Source: CAD feature listing. Evaluate the final solid. Frame: model axes, mm. A direction names the side the tool comes from. Give positions to 0.01 mm unless a question says otherwise; leave off trailing zeros. Loops run counter-clockwise (first coordinate to the right, second up) from the corner with the lowest first, then second, coordinate; pieces in that order, holes last. Notation, with made-up numbers: (46, 40.5) - (92, 40.5) arc R5 ccw to (92, 45.5) - close; hole circle Ø1 at (59.5, 62). An arc over 180 degrees is marked (long way). Write each question's results on one line, items separated by ' | '. Start each with the question number.
(1) Cut plane B-B on y = -8. Return the cut outline in (x, z).
(2) Contact query for flat-ended pins moving along their axis: pin 1 (2 mm diameter, centred on y = -1, z = -9.5, fed in from -X); pin 2 (5 mm diameter, centred on x = 8.5, z = -1, fed in from -Y); pin 3 (1.5 mm diameter, centred on x = 3, y = -1.5, fed in from +Z); pin 4 (4 mm diameter, centred on x = 3.5, y = -10, fed in from +Z). Output: stop coordinate, or through.
(3) Cut plane D-D on z = -6. Return the cut outline in (x, y).
(4) Reachability of faces 5 (the cylindrical face through (0.8, -0.95, 10.75)), 6 (the cylindrical face through (2.937, 0.056, 12.834)) from +Z, -Z, +X, -X, +Y, -Y: full face, straight path, thin tool, end or side. Return the list, or none.
(5) Pull-direction query (X, two-part tool) for faces 1 (the cylindrical face through (11.851, 1.972, -1.223)), 2 (the flat face through (4, -4, 0)), 3 (the flat face through (0, -9, 0)), 4 (the flat face through (-2.5, 2, 0.2)); classes: pulls with the +X half, pulls with the -X half, needs draft (parallel to the pull), parting line crosses it, or undercut.
(6) Cut plane A-A on z = 0. Return the cut outline in (x, y) (3 decimals), then the cut area to 3 significant figures.
(7) Cut plane C-C on x = 13. Return the cut outline in (y, z), then the cut area to 3 significant figures.
(8) Material intervals for line 1 along Z through (x, y) = (-1, -1); line 2 along Y through (x, z) = (-1.3, -5); line 3 along X through (y, z) = (0.9, 0), sorted ascending. Write a range as [from, to].
from build123d import *

# Parameters (mm, degrees)
BOSS_EXTRUDE1_DEPTH       = 4
FILLET1_R                 = 8
SKETCH7_W                 = 3
SKETCH7_H                 = 26
BOSS_EXTRUDE3_DEPTH       = 15.5
M3X0_5_TAPPED_HOLE1_D     = 2.5
M3X0_5_TAPPED_HOLE1_DEPTH = 7.5
M3X0_5_TAPPED_HOLE1_TIP   = 0.751075774
M3_CLEARANCE_HOLE2_D      = 3.4
SKETCH12_W                = 1
SKETCH12_H                = 26
BOSS_EXTRUDE4_DEPTH       = 2
FILLET4_R                 = 6
FILLET5_R                 = 1
FILLET6_R                 = 5
FILLET7_R                 = 0.25
CHAMFER1_SIZE             = 1
CHAMFER2_SIZE             = 0.5


with BuildPart() as part:
    # Sketch1 → Boss-Extrude1 (new, symmetric)
    with BuildSketch(Plane(origin=(0, 0, 0), x_dir=(1, 0, 0), z_dir=(0, 1, 0))):
        Polygon((0, 0), (0, 13), (3, 13), (25.516660498, 0), (3, -13), (0, -13), align=None)
    extrude(amount=BOSS_EXTRUDE1_DEPTH, both=True)

    # Fillet1
    fillet1_edges = [part.edges().sort_by_distance(p)[0] for p in [
        (25.516660498, 0, 0),
    ]]
    fillet(fillet1_edges, radius=FILLET1_R)

    # Sketch7 → Boss-Extrude3 (add)
    with BuildSketch(Plane(origin=(0, 2.5, 0), x_dir=(1, 0, 0), z_dir=(0, 1, 0))):
        with Locations((-1.5, 0)):
            Rectangle(SKETCH7_W, SKETCH7_H)
    extrude(amount=-BOSS_EXTRUDE3_DEPTH)

    # M3x0.5 Tapped Hole1
    with Locations(Plane.ZY.offset(3)):
        with Locations((9.5, -1), (-9.5, -1)):
            Hole(M3X0_5_TAPPED_HOLE1_D / 2, depth=M3X0_5_TAPPED_HOLE1_DEPTH)
            with Locations((0, 0, -(M3X0_5_TAPPED_HOLE1_DEPTH + M3X0_5_TAPPED_HOLE1_TIP / 2))):  # 118° drill point
                Cone(0, M3X0_5_TAPPED_HOLE1_D / 2, M3X0_5_TAPPED_HOLE1_TIP, mode=Mode.SUBTRACT)

    # M3 Clearance Hole2 (through all)
    with Locations(Plane.ZY.offset(3)):
        with Locations((-5, -8), (5, -8)):
            Hole(M3_CLEARANCE_HOLE2_D / 2)

    # Sketch12 → Boss-Extrude4 (add)
    with BuildSketch(Plane(origin=(0, 4, 0), x_dir=(1, 0, 0), z_dir=(0, 1, 0))):
        with Locations((-0.5, 0)):
            Rectangle(SKETCH12_W, SKETCH12_H)
    extrude(amount=-BOSS_EXTRUDE4_DEPTH)

    # Sketch20 → CBORE for M5 SHCS1 (revolve, cut)
    with BuildSketch(Plane(origin=(9.5, -4, 0), x_dir=(0, 0, -1), z_dir=(1, 0, 0))):
        Polygon((0, 0), (0, 8), (2.675, 8), (2.65, 7.975), (2.65, 4.025), (2.675, 4), (5, 4), (5, 0), align=None)
    revolve(axis=Axis((9.5, -10.35, 0), (0, 1, 0)), mode=Mode.SUBTRACT)

    # Fillet4
    fillet4_edges = [part.edges().sort_by_distance(p)[0] for p in [
        (-1.5, -13, 13),
        (-1.5, -13, -13),
    ]]
    fillet(fillet4_edges, radius=FILLET4_R)

    # Fillet5
    fillet5_edges = [part.edges().sort_by_distance(p)[0] for p in [
        (0, -4, 0),
    ]]
    fillet(fillet5_edges, radius=FILLET5_R)

    # Fillet6
    fillet6_edges = [part.edges().sort_by_distance(p)[0] for p in [
        (3, 0, -13),
        (3, 0, 13),
    ]]
    fillet(fillet6_edges, radius=FILLET6_R)

    # Fillet7
    fillet7_edges = [part.edges().sort_by_distance(p)[0] for p in [
        (-1, 2.5, 0),
    ]]
    fillet(fillet7_edges, radius=FILLET7_R)

    # Chamfer1
    chamfer1_edges = [part.edges().sort_by_distance(p)[0] for p in [
        (-3, 2.5, 0),
    ]]
    chamfer(chamfer1_edges, length=CHAMFER1_SIZE)

    # Chamfer2
    chamfer2_edges = [part.edges().sort_by_distance(p)[0] for p in [
        (-1, 4, 0),
    ]]
    chamfer(chamfer2_edges, length=CHAMFER2_SIZE)


solid = part.part
Ans:
1) outline: (-3, -12.92) - (0, -12.92) - (0, -6.7) - (-3, -6.7) - close; (-3, -3.3) - (0, -3.3) - (0, 3.3) - (-3, 3.3) - close; (-3, 6.7) - (0, 6.7) - (0, 12.92) - (-3, 12.92) - close
2) pin 1: x = 4.65 | pin 2: y = 0 | pin 3: z = 12.97 | pin 4: through
3) outline: (-3, -13) - (0, -13) - (0, -9.37) - (-3, -9.37) - close; (-3, -6.63) - (0, -6.63) - (0, -5) arc R1 cw to (1, -4) - (14.81, -4) - (14.81, 4) - (-0.5, 4) - (-1, 3.5) - (-1, 2.75) arc R0.25 cw to (-1.25, 2.5) - (-2, 2.5) - (-3, 1.5) - close
4) face 5: -X | face 6: +Z, +X, +Y, -Y
5) face 1: undercut | face 2: needs draft | face 3: pulls with the +X half | face 4: pulls with the -X half
6) outline: (-3, -13) - (0, -13) - (0, -5) arc R1 cw to (1, -4) - (4.5, -4) - (4.5, 0) - (6.825, 0) - (6.85, 0.025) - (6.85, 3.975) - (6.825, 4) - (-0.5, 4) - (-1, 3.5) - (-1, 2.75) arc R0.25 cw to (-1.25, 2.5) - (-2, 2.5) - (-3, 1.5) - close; (12.15, 0.025) - (12.175, 0) - (14.5, 0) - (14.5, -4) - (17.517, -4) - (17.517, 4) - (12.175, 4) - (12.15, 3.975) - close | area: 127 mm^2
7) outline: (-4, -7.23) - (4, -7.23) - (4, 7.23) - (-4, 7.23) - (-4, 3.57) - (0, 3.57) - (0, -3.57) - (-4, -3.57) - close | area: 87.1 mm^2
8) line 1: [-13, -10.75], [-8.25, 8.25], [10.75, 13] | line 2: [-13, -9.7], [-6.3, 2.5] | line 3: [-3, 6.85], [12.15, 17.52]
